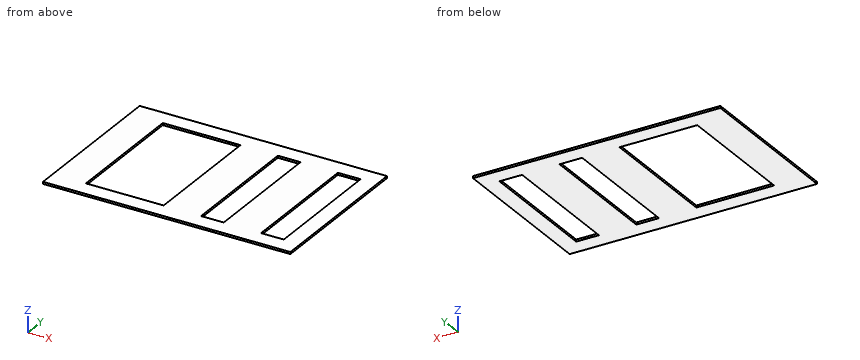
```python
from build123d import *

# Parameters (mm, degrees)
SKETCH_W   = 762
SKETCH_H   = 495.3
SKETCH_W_2 = 70
SKETCH_H_2 = 393.7
SKETCH_W_3 = 239.6
PAD_DEPTH  = 6.35


with BuildPart() as part:
    # Sketch → Pad (new body)
    with BuildSketch(Plane.XY.offset(6.35)):
        Rectangle(SKETCH_W, SKETCH_H)
        with Locations((295.2, 0)):
            Rectangle(SKETCH_W_2, SKETCH_H_2, mode=Mode.SUBTRACT)
        with Locations((-159.6, 0)):
            Rectangle(SKETCH_W_3, SKETCH_H_2, mode=Mode.SUBTRACT)
        with Locations((110.2, 0)):
            Rectangle(SKETCH_W_2, SKETCH_H_2, mode=Mode.SUBTRACT)
    extrude(amount=PAD_DEPTH)


solid = part.part
```
Read the model definition and answer for the solid it produces. Units are mm, in the model's axes. Coordinates: 2 decimals unless noted, no trailing zeros. Write each loop counter-clockwise with the first axis right and the second up, starting at its lowest first coordinate (ties: lowest second). Pieces come first, ordered by that corner, then holes. Notation, with made-up numbers: (75.25, 72) - (121.25, 72) arc R24 ccw to (121.25, 93) - close; hole circle Ø11 at (-11, -1.5). An arc over 180 degrees is marked (long way). Answer as a JSON object with one key per item and string values. Group by question number.
1. A cutting plane is placed at B-B (y = -54). Determine the outline of the cut face in (x, z).
2. Consider L1, parallel to X at y = -32, z = 7.5; L2, parallel to Y at x = -41, z = 7. Determine where each line is inside the solid, lowest interval first. Write a range as [from, to].
3. A cutting plane is placed at A-A (x = 298). Determine the outline of the cut face in (y, z).
4. A cutting plane is placed at C-C (z = 11.5). Determine the outline of the cut face in (x, y), plus the area to 3 significant figures.
Worked out:
{
 "1": {"outline": "(-381, 6.35) - (-279.4, 6.35) - (-279.4, 12.7) - (-381, 12.7) - close; (-39.8, 6.35) - (75.2, 6.35) - (75.2, 12.7) - (-39.8, 12.7) - close; (145.2, 6.35) - (260.2, 6.35) - (260.2, 12.7) - (145.2, 12.7) - close; (330.2, 6.35) - (381, 6.35) - (381, 12.7) - (330.2, 12.7) - close"},
 "2": {"L1": "x = [-381, -279.4], [-39.8, 75.2], [145.2, 260.2], [330.2, 381]", "L2": "y = [-247.65, -196.85], [196.85, 247.65]"},
 "3": {"outline": "(-247.65, 6.35) - (-196.85, 6.35) - (-196.85, 12.7) - (-247.65, 12.7) - close; (196.85, 6.35) - (247.65, 6.35) - (247.65, 12.7) - (196.85, 12.7) - close"},
 "4": {"outline": "(-381, -247.65) - (381, -247.65) - (381, 247.65) - (-381, 247.65) - close; hole (-279.4, -196.85) - (-39.8, -196.85) - (-39.8, 196.85) - (-279.4, 196.85) - close; hole (75.2, -196.85) - (145.2, -196.85) - (145.2, 196.85) - (75.2, 196.85) - close; hole (260.2, -196.85) - (330.2, -196.85) - (330.2, 196.85) - (260.2, 196.85) - close", "area": "228,000 mm²"}
}
